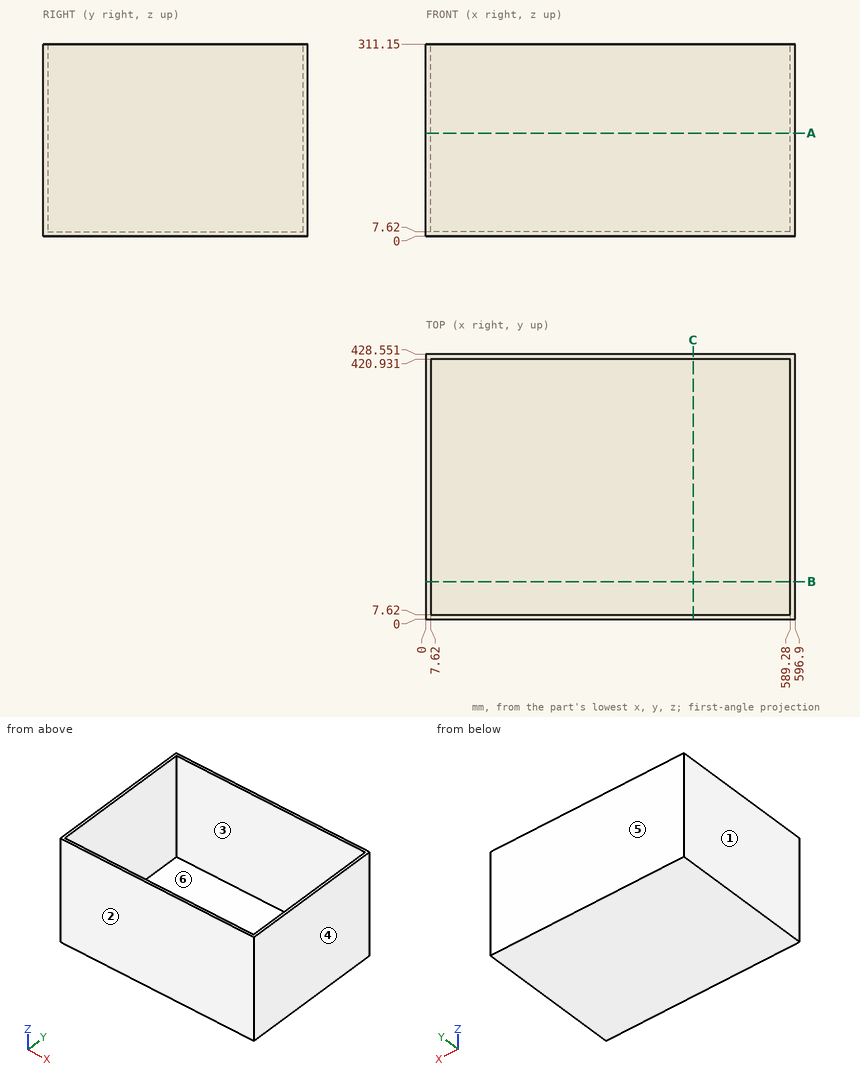
Geometry: see drawing. Coordinates: mm, zero at the bounding-box minimum. A direction names the side the tool comes from. Coordinates: 2 decimals unless noted, no trailing zeros. Order: outer loops, then holes, each group sorted by start corner. A loop starts at its lowest first (then second) coordinate and runs counter-clockwise, first axis right, second up. Notation, with made-up numbers: M -21.75,39.25 L -14.75,39.25 A27 ccw -14.75,68.25 Z; hole C 53,-33 d6. An arc over 180 degrees is marked long. Write item = value, one per line. Start each with the question number.
(1) Section C-C on x = 432. Output: boundary loops of the cut face in (y, z), and give its area (3 significant figures).
(2) Pull-direction query (X, two-part tool) for the marked faces 1, 2, 3 and 4; classes: released by +X, released by -X, zero draft, split by the parting line, or undercut.
(3) Reachability of the marked faces 5 and 6 from +Z, -Z, +X, -X, +Y, -Y: full face, straight path, thin tool, end or side. Return the list, or none.
(4) Section B-B on y = 61. Output: boundary loops of the cut face in (x, z).
(5) First-contact query: P1, Ø6, axis at x = 159.5, y = 124.5, coming from the +Z side. Flat tip, straight axial feed; report the tip coordinate or a pass-through.
(6) Section A-A on z = 167. Output: boundary loops of the cut face in (x, y), and give its area (3 significant figures).
(7) Line query: line 1 along X through (y, z) = (374, 108.5); line 2 along Y through (x, z) = (312, 231.5); line 3 along Z through (x, y) = (453.5, 330.5). Output: solid intervals per line, ascending. Write a range as [from, to].
Result set:
q1.outline = M 0,0 L 428.55,0 L 428.55,311.15 L 420.93,311.15 L 420.93,7.62 L 7.62,7.62 L 7.62,311.15 L 0,311.15 Z
q1.area = 7,890 mm²
q2.face_1 = released by -X
q2.face_2 = zero draft
q2.face_3 = undercut
q2.face_4 = released by +X
q3.face_5 = +Z, -Z, +X, -X, +Y
q3.face_6 = +Z
q4.outline = M 0,0 L 596.9,0 L 596.9,311.15 L 589.28,311.15 L 589.28,7.62 L 7.62,7.62 L 7.62,311.15 L 0,311.15 Z
q5.P1 = 7.62
q6.outline = M 0,0 L 596.9,0 L 596.9,428.55 L 0,428.55 Z; hole M 7.62,7.62 L 589.28,7.62 L 589.28,420.93 L 7.62,420.93 Z
q6.area = 15,400 mm²
q7.line_1 = [0, 7.62], [589.28, 596.9]
q7.line_2 = [0, 7.62], [420.93, 428.55]
q7.line_3 = [0, 7.62]
